Part print with two shaded views. Sizes in mm from the minimum x, y, z corner. A direction names the side the tool comes from. Give positions to 0.01 mm unless a question says otherwise; leave off trailing zeros. Order: outer loops, then holes, each group sorted by start corner. A loop starts at its lowest first (then second) coordinate and runs counter-clockwise, first axis right, second up. Notation, with made-up numbers: M 28,83 L 37,83 A12 ccw 37,90 Z; hole C -34.75,12.5 d8. An arc over 180 degrees is marked long. Return JSON: item names as keys, results as strings.
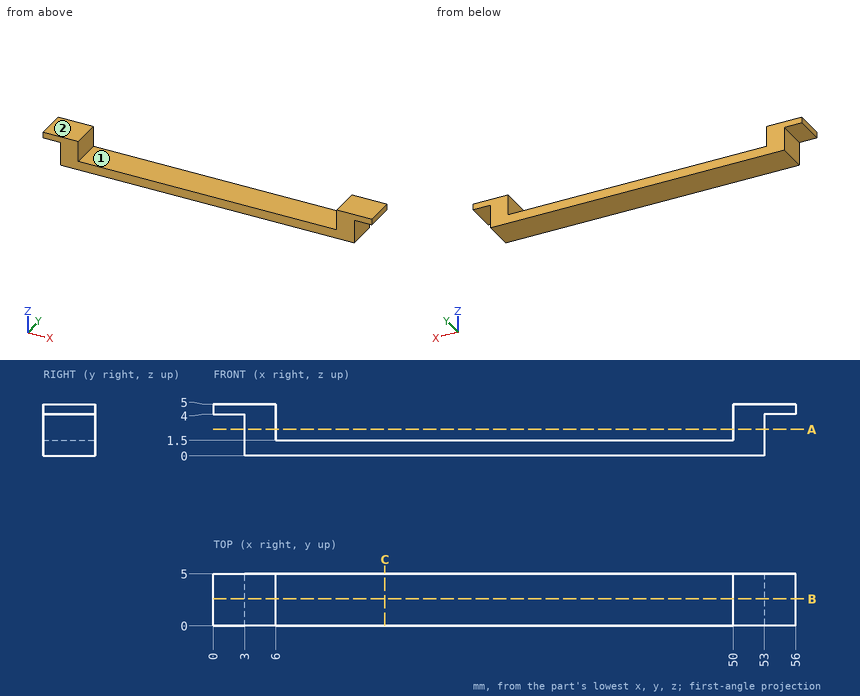
Q1. Pin check, flat tips, straight feed: pin 1 (1.5 mm diameter, centred on x = 54.5, y = 2, fed in from -Z); pin 2 (2 mm diameter, centred on y = 1.5, z = 2, fed in from +X); pin 3 (2.5 mm diameter, centred on x = 27, y = 2, fed in from +Z); pin 4 (3 mm diameter, centred on x = 44, y = 3, fed in from -Z). Stop position of each tip, or through.
Established:
{"pin 1": "stops at z = 4", "pin 2": "stops at x = 53", "pin 3": "stops at z = 1.5", "pin 4": "stops at z = 0"}
Q2. Probe line 1 along X through (y, z) = (4.6, 4.6); line 2 along X through (y, z) = (0.85, 2.75); line 3 along Z through (x, y) = (7, 2.7). List the from-to ranges inside material, lowest first.
Established:
{"line 1": "x = 0 to 6, 50 to 56", "line 2": "x = 3 to 6, 50 to 53", "line 3": "z = 0 to 1.5"}
Q3. Band-saw the part on C-C (x = 16.5). Give the cut face in (y, z).
Established:
{"outline": "M 0,0 L 5,0 L 5,1.5 L 0,1.5 Z"}
Q4. Band-saw the part on B-B (y = 2.6). Give the cut face in (x, z), then the cut area to 3 significant figures.
Established:
{"outline": "M 0,4 L 3,4 L 3,0 L 53,0 L 53,4 L 56,4 L 56,5 L 50,5 L 50,1.5 L 6,1.5 L 6,5 L 0,5 Z", "area": "102 mm²"}
Q5. Band-saw the part on A-A (z = 2.55). Give the cut face in (x, y), then the cut area to 3 significant figures.
Established:
{"outline": "M 3,0 L 6,0 L 6,5 L 3,5 Z; M 50,0 L 53,0 L 53,5 L 50,5 Z", "area": "30.0 mm²"}
Q6. 3-axis set-ups, long thin cutter, end or side, ignore diameter. For the marked faces 1 and 2: which of +Z, -Z, +X, -X, +Y, -Y reach the whole face in a straight line?
Established:
{"face 1": "+Z, +Y, -Y", "face 2": "+Z, +X, -X, +Y, -Y"}
